```python
from build123d import *

# Parameters (mm, degrees)
SKETCH1_W           = 57
SKETCH1_H           = 100
BOSS_EXTRUDE1_DEPTH = 80
SKETCH3_W           = 75
SKETCH3_H           = 90
CUT_EXTRUDE1_DEPTH  = 52
SKETCH4_R           = 4.025
CUT_EXTRUDE2_DEPTH  = 114.213294272
BOSS_EXTRUDE2_DEPTH = 30
CUT_EXTRUDE5_REACH  = 112.223
SKETCH8_W           = 90
SKETCH8_H           = 40
SKETCH5_R           = 11
CUT_EXTRUDE3_DEPTH  = 141.791512528


with BuildPart() as part:
    # Sketch1 → Boss-Extrude1 (new body)
    with BuildSketch(Plane(origin=(0, 0, 0), x_dir=(1, 0, 0), z_dir=(0, 1, 0))):
        Rectangle(SKETCH1_W, SKETCH1_H)
    extrude(amount=BOSS_EXTRUDE1_DEPTH)

    # Sketch3 → Cut-Extrude1 (cut)
    with BuildSketch(Plane(origin=(28.5, 40, 0), x_dir=(0, 1, 0), z_dir=(-1, 0, 0))):
        with Locations((2.5, 0)):
            Rectangle(SKETCH3_W, SKETCH3_H)
    extrude(amount=CUT_EXTRUDE1_DEPTH, mode=Mode.SUBTRACT)

    # Sketch4 → Cut-Extrude2 (cut, through all)
    with BuildSketch(Plane(origin=(-40, 5, 0), x_dir=(-1, 0, 0), z_dir=(0, -1, 0))):
        with Locations(Location((-40, 0, 0), (0, 0, 90))):
            Circle(SKETCH4_R)
    extrude(amount=CUT_EXTRUDE2_DEPTH, mode=Mode.SUBTRACT)

    # Sketch7 → Boss-Extrude2 (add)
    with BuildSketch(Plane.ZY.offset(28.5)):
        Polygon((-50, 80), (-45, 80), (-45, 40), (45, 40), (45, 80), (50, 80), (50, 35), (-50, 35), align=None)
    extrude(amount=BOSS_EXTRUDE2_DEPTH)

    # Sketch8 → Cut-Extrude5 (cut, up to next)
    with BuildSketch(Plane.ZY.offset(28.5), mode=Mode.PRIVATE) as cut_extrude5_sk1:
        with Locations((0, 60)):
            Rectangle(SKETCH8_W, SKETCH8_H)
    cut_extrude5_tool1 = extrude(cut_extrude5_sk1.sketch, amount=-CUT_EXTRUDE5_REACH, mode=Mode.PRIVATE) & part.part
    add(cut_extrude5_tool1.solids().sort_by_distance((-28.5, 60, 0))[0], mode=Mode.SUBTRACT)

    # Sketch5 → Cut-Extrude3 (cut, through all)
    with BuildSketch(Plane(origin=(0, 0, -50), x_dir=(-1, 0, 0), z_dir=(0, 0, -1))):
        with Locations((43.5, 62.5)):
            Circle(SKETCH5_R)
        with BuildLine():
            Line((-22.1, 59.6), (-16.1, 59.6))
            ThreePointArc((-16.1, 59.6), (-14.6, 58.1), (-16.1, 56.6))
            Line((-16.1, 56.6), (-22.1, 56.6))
            ThreePointArc((-22.1, 56.6), (-23.6, 58.1), (-22.1, 59.6))
        make_face()
        with BuildLine():
            Line((-0.5, 31), (-6.5, 31))
            ThreePointArc((-6.5, 31), (-18, 42.5), (-6.5, 54))
            Line((-6.5, 54), (-0.5, 54))
            ThreePointArc((-0.5, 54), (11, 42.5), (-0.5, 31))
        make_face()
        with BuildLine():
            Line((-22.1, 25.4), (-16.1, 25.4))
            ThreePointArc((-16.1, 25.4), (-14.6, 26.9), (-16.1, 28.4))
            Line((-16.1, 28.4), (-22.1, 28.4))
            ThreePointArc((-22.1, 28.4), (-23.6, 26.9), (-22.1, 25.4))
        make_face()
        with BuildLine():
            Line((15.1, 25.4), (9.1, 25.4))
            ThreePointArc((9.1, 25.4), (7.6, 26.9), (9.1, 28.4))
            Line((9.1, 28.4), (15.1, 28.4))
            ThreePointArc((15.1, 28.4), (16.6, 26.9), (15.1, 25.4))
        make_face()
        with BuildLine():
            Line((15.1, 59.6), (9.1, 59.6))
            ThreePointArc((9.1, 59.6), (7.6, 58.1), (9.1, 56.6))
            Line((9.1, 56.6), (15.1, 56.6))
            ThreePointArc((15.1, 56.6), (16.6, 58.1), (15.1, 59.6))
        make_face()
    extrude(amount=-CUT_EXTRUDE3_DEPTH, mode=Mode.SUBTRACT)


solid = part.part
```
Input: part model. Units: mm. Frame: model coordinates. A direction names the side the tool comes from. Give positions to 0.01 mm unless a question says otherwise; leave off trailing zeros. Order: outer loops, then holes, each group sorted by start corner. A loop starts at its lowest first (then second) coordinate and runs counter-clockwise, first axis right, second up. Notation, with made-up numbers: (3.5, 37.25) -> (41.5, 37.25) arc R18 cw to (41.5, 68.25) -> close; hole circle Ø3 at (39.5, -1). An arc over 180 degrees is marked (long way). Write each question's results on one line, items separated by ' | '. Start each with the question number.
Item 1: Cut plane B-B on x = -43.5. Return the cut outline in (y, z).
Item 2: Cut plane C-C on y = 15. Return the cut outline in (x, z).
Item 3: Mould query, pull axis X, two halves, no side actions, for faces 1 (the cylindrical face through (-7.6, 58.1, -47.5)), 2 (the cylindrical face through (-16.6, 26.9, -47.5)), 3 (the flat face through (28.5, 4, 4)), 4 (the flat face through (-41, 40, -1)). Classes: pulls with the +X half, pulls with the -X half, needs draft (parallel to the pull), parting line crosses it, or undercut.
Item 4: Set-up query: faces 5 (the flat face through (-14, 80, 47)), 6 (the cylindrical face through (-16.6, 58.1, -47.5)), 7 (the flat face through (-43, 35, 1)). Return all of +Z, -Z, +X, -X, +Y, -Y with unobstructed straight access to the full face (end or side cutting, diameter ignored); none if empty.
Item 5: Cut plane A-A on y = 42.5. Return the cut outline in (x, z).
Item 6: Line query: line 1 (Z direction, x = 0, y = 2.75) (3 decimals); line 2 (Z direction, x = -15, y = 74); line 3 (Y direction, x = -43.5, z = -47.9). Output: solid intervals per line, ascending.
Item 7: Contact query for flat-ended pins moving along their axis: P1, Ø3, axis at x = -31, z = -10.5, coming from the +Y side; P2, Ø10, axis at y = 28.5, z = -34.5, coming from the -X side; P3, Ø1, axis at x = -2, z = -8, coming from the +Y side. Output: stop coordinate, or through.
Item 8: Cut plane D-D on z = -20. Return the cut outline in (x, y).
Established:
1) outline: (35, -50) -> (51.5, -50) -> (51.5, -45) -> (40, -45) -> (40, 45) -> (51.5, 45) -> (51.5, 50) -> (35, 50) -> close; (73.5, -50) -> (80, -50) -> (80, -45) -> (73.5, -45) -> close; (73.5, 45) -> (80, 45) -> (80, 50) -> (73.5, 50) -> close
2) outline: (-28.5, -50) -> (28.5, -50) -> (28.5, -45) -> (-23.5, -45) -> (-23.5, 45) -> (28.5, 45) -> (28.5, 50) -> (-28.5, 50) -> close
3) face 1: undercut | face 2: undercut | face 3: pulls with the +X half | face 4: needs draft
4) face 5: +Z, -Z, +X, -X, +Y | face 6: +Z, -Z | face 7: +Z, -Z, -X, -Y
5) outline: (-58.5, -50) -> (-11, -50) -> (-11, -45) -> (-58.5, -45) -> close; (-58.5, 45) -> (-11, 45) -> (-11, 50) -> (-58.5, 50) -> close; (18, -50) -> (28.5, -50) -> (28.5, -45) -> (18, -45) -> close; (18, 45) -> (28.5, 45) -> (28.5, 50) -> (18, 50) -> close
6) line 1: -50 to -4.025, 4.025 to 50 | line 2: -50 to -45, 45 to 50 | line 3: 35 to 51.5, 73.5 to 80
7) P1: y = 40 | P2: x = -28.5 | P3: y = 5
8) outline: (-58.5, 35) -> (-28.5, 35) -> (-28.5, 0) -> (28.5, 0) -> (28.5, 5) -> (-23.5, 5) -> (-23.5, 40) -> (-58.5, 40) -> close
